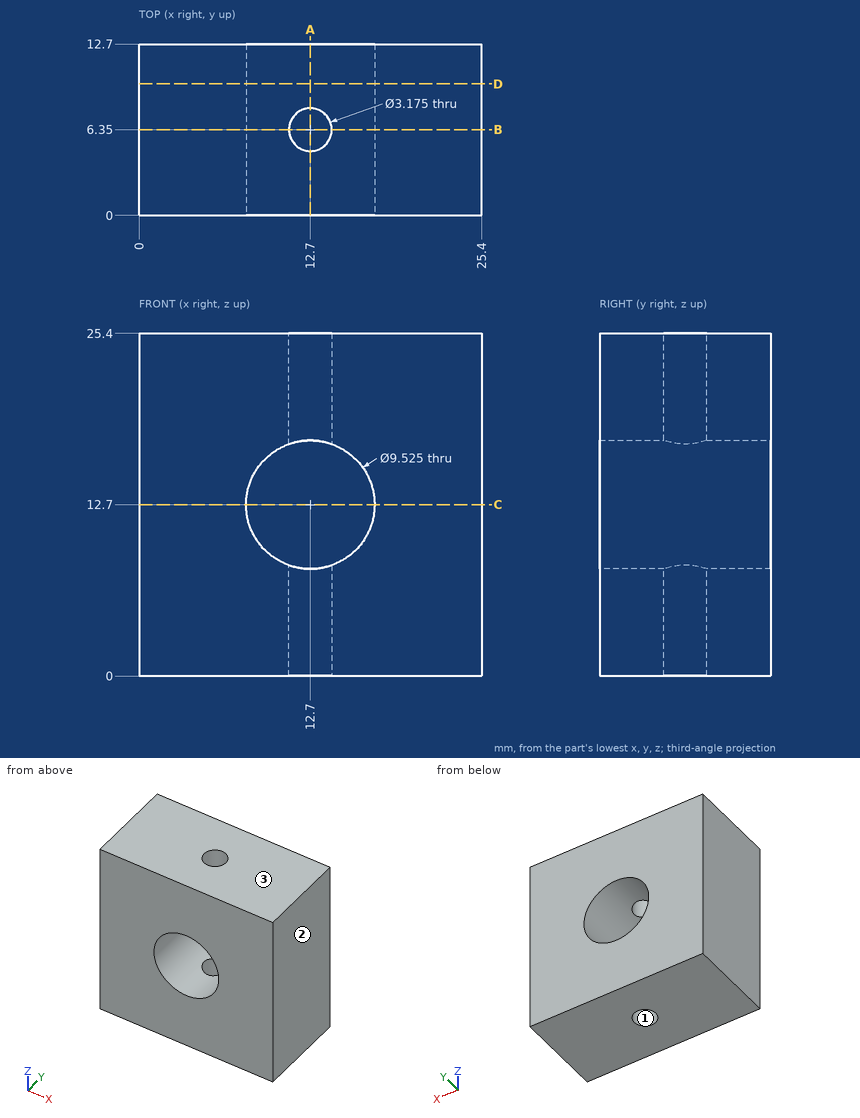
Print and shaded views of the part. All mm, measured from the part's lowest x, y and z. Round coordinates to 2 decimals unless told otherwise and drop trailing zeros. Write each loop counter-clockwise with the first axis right and the second up, starting at its lowest first coordinate (ties: lowest second). Pieces come first, ordered by that corner, then holes. Notation, with made-up numbers: (-23, -33.75) - (-5, -33.75) arc R19 cw to (-5, -29.75) - close; hole circle Ø2 at (59, -16.75). An arc over 180 degrees is marked (long way). Write each question's results on one line, items separated by ' | '. Start each with the question number.
Item 1: Saw through at D-D (y = 9.75). Write the cut outline in (x, z) (1 decimal).
Item 2: Wall check: L1, parallel to Y at x = 12.7, z = 6.75; L2, parallel to X at y = 8.25, z = 12.5; L3, parallel to X at y = 6.5, z = 23.75. Give the ranges that are in metal, low to high. Write a range as [from, to].
Item 3: Saw through at C-C (z = 12.7). Write the cut outline in (x, y).
Item 4: Saw through at A-A (x = 12.7). Write the cut outline in (y, z).
Item 5: Mould opens along X. For the marked faces 1, 2 and 3 say: pulls with the +X half, pulls with the -X half, needs draft (parallel to the pull), parting line crosses it, or undercut.
Item 6: Saw through at B-B (y = 6.35). Write the cut outline in (x, z) (1 decimal).
Results are:
1) outline: (0, 0) - (25.4, 0) - (25.4, 25.4) - (0, 25.4) - close; hole circle Ø9.5 at (12.7, 12.7)
2) L1: y = [0, 4.76], [7.94, 12.7] | L2: x = [0, 7.94], [17.46, 25.4] | L3: x = [0, 11.12], [14.28, 25.4]
3) outline: (0, 0) - (7.94, 0) - (7.94, 12.7) - (0, 12.7) - close; (17.46, 0) - (25.4, 0) - (25.4, 12.7) - (17.46, 12.7) - close
4) outline: (0, 0) - (4.76, 0) - (4.76, 7.94) - (0, 7.94) - close; (0, 17.46) - (4.76, 17.46) - (4.76, 25.4) - (0, 25.4) - close; (7.94, 0) - (12.7, 0) - (12.7, 7.94) - (7.94, 7.94) - close; (7.94, 17.46) - (12.7, 17.46) - (12.7, 25.4) - (7.94, 25.4) - close
5) face 1: undercut | face 2: pulls with the +X half | face 3: needs draft
6) outline: (0, 0) - (11.1, 0) - (11.1, 8.2) arc R4.8 cw to (11.1, 17.2) - (11.1, 25.4) - (0, 25.4) - close; (14.3, 0) - (25.4, 0) - (25.4, 25.4) - (14.3, 25.4) - (14.3, 17.2) arc R4.8 cw to (14.3, 8.2) - close
